```python
from build123d import *

# Parameters (mm, degrees)
SKETCH1_W           = 199
SKETCH1_H           = 129.3
SKETCH1_R           = 7.9
SKETCH1_R_2         = 3.5
SKETCH1_W_2         = 2.6
SKETCH1_H_2         = 1.1
BOSS_EXTRUDE1_DEPTH = 2.13


with BuildPart() as part:
    # Sketch1 → Boss-Extrude1 (new body)
    with BuildSketch(Plane(origin=(0, 0, 0), x_dir=(1, 0, 0), z_dir=(0, 1, 0))):
        Rectangle(SKETCH1_W, SKETCH1_H)
        with Locations((-70, 45)):
            Circle(SKETCH1_R, mode=Mode.SUBTRACT)
        with Locations((-35, 45)):
            Circle(SKETCH1_R, mode=Mode.SUBTRACT)
        with Locations((0, 45)):
            Circle(SKETCH1_R, mode=Mode.SUBTRACT)
        with Locations((35, 45)):
            Circle(SKETCH1_R, mode=Mode.SUBTRACT)
        with Locations((-35, 15)):
            Circle(SKETCH1_R, mode=Mode.SUBTRACT)
        with Locations((0, 15)):
            Circle(SKETCH1_R, mode=Mode.SUBTRACT)
        with Locations((35, 15)):
            Circle(SKETCH1_R, mode=Mode.SUBTRACT)
        with Locations((-35, -15)):
            Circle(SKETCH1_R, mode=Mode.SUBTRACT)
        with Locations((0, -15)):
            Circle(SKETCH1_R, mode=Mode.SUBTRACT)
        with Locations((35, -15)):
            Circle(SKETCH1_R, mode=Mode.SUBTRACT)
        with Locations((-35, -45)):
            Circle(SKETCH1_R, mode=Mode.SUBTRACT)
        with Locations((0, -45)):
            Circle(SKETCH1_R, mode=Mode.SUBTRACT)
        with Locations((35, -45)):
            Circle(SKETCH1_R, mode=Mode.SUBTRACT)
        with Locations((-70, 15)):
            Circle(SKETCH1_R, mode=Mode.SUBTRACT)
        with Locations((-70, -15)):
            Circle(SKETCH1_R, mode=Mode.SUBTRACT)
        with Locations((-70, -45)):
            Circle(SKETCH1_R, mode=Mode.SUBTRACT)
        with Locations((70, 35)):
            Circle(SKETCH1_R_2, mode=Mode.SUBTRACT)
        with Locations((70, 0)):
            Circle(SKETCH1_R_2, mode=Mode.SUBTRACT)
        with Locations((70, -35)):
            Circle(SKETCH1_R_2, mode=Mode.SUBTRACT)
        with Locations((70, 43.05)):
            Rectangle(SKETCH1_W_2, SKETCH1_H_2, mode=Mode.SUBTRACT)
        with Locations((70, 8.05)):
            Rectangle(SKETCH1_W_2, SKETCH1_H_2, mode=Mode.SUBTRACT)
        with Locations((70, -26.95)):
            Rectangle(SKETCH1_W_2, SKETCH1_H_2, mode=Mode.SUBTRACT)
    extrude(amount=BOSS_EXTRUDE1_DEPTH)


solid = part.part
```
Design review of the part built by this model. Coordinates are the model's own, in mm. Coordinates: 2 decimals unless noted, no trailing zeros. Order: outer loops, then holes, each group sorted by start corner. A loop starts at its lowest first (then second) coordinate and runs counter-clockwise, first axis right, second up.
1) Mouldability with a two-part tool opening along Z and no side actions: class faces 1 (the flat face through (-1, 0, -1)), 2 (the cylindrical face through (-62.702, 1.05, -41.974)) as +Z half, -Z half, draft (parallel to the pull), parting line (faces both ways), or undercut.
2) Take a section at A-A, the plane x = -70. Give the boundary of the cut face in (y, z).
3) Wall thickness on line 1 along Z through (x, y) = (-35, 1.05); line 2 along X through (y, z) = (1.35, -45); line 3 along Z through (x, y) = (41.5, 0.4): over which ranges is each line inside the solid? List them lowest first.
4) Take a section at C-C, the plane y = 0.4. State how many separate pieces and enclosed holes the cut face has, and give its area (3 significant figures).
5) Take a section at B-B, the plane z = -15. Give the boundary of the cut face in (x, y).
Returned:
1. face 1: draft
1. face 2: undercut
2. outline: (0, -64.65) - (2.13, -64.65) - (2.13, -52.9) - (0, -52.9) - close; (0, -37.1) - (2.13, -37.1) - (2.13, -22.9) - (0, -22.9) - close; (0, -7.1) - (2.13, -7.1) - (2.13, 7.1) - (0, 7.1) - close; (0, 22.9) - (2.13, 22.9) - (2.13, 37.1) - (0, 37.1) - close; (0, 52.9) - (2.13, 52.9) - (2.13, 64.65) - (0, 64.65) - close
3. line 1: z = -64.65 to -52.9, -37.1 to -22.9, -7.1 to 7.1, 22.9 to 37.1, 52.9 to 64.65
3. line 2: x = -99.5 to -77.9, -62.1 to -42.9, -27.1 to -7.9, 7.9 to 27.1, 42.9 to 99.5
3. line 3: z = -64.65 to -49.49, -40.51 to -19.49, -10.51 to 10.51, 19.49 to 40.51, 49.49 to 64.65
4. separate pieces: 1
4. enclosed holes: 22
4. area: 22,500 mm2
5. outline: (-99.5, 0) - (-77.9, 0) - (-77.9, 2.13) - (-99.5, 2.13) - close; (-62.1, 0) - (-42.9, 0) - (-42.9, 2.13) - (-62.1, 2.13) - close; (-27.1, 0) - (-7.9, 0) - (-7.9, 2.13) - (-27.1, 2.13) - close; (7.9, 0) - (27.1, 0) - (27.1, 2.13) - (7.9, 2.13) - close; (42.9, 0) - (99.5, 0) - (99.5, 2.13) - (42.9, 2.13) - close
